```python
from build123d import *

# Parameters (mm, degrees)
F0_W     = 45
F0_H     = 100
F1_DEPTH = 10
F2_W     = 17
F2_H     = 100
F3_DEPTH = 8.5
F4_W     = 34
F4_H     = 100
F5_DEPTH = 7
F8_R     = 16.5
F9_DEPTH = 10


with BuildPart() as f1:
    # F0 (on Top) → F1 (new body)
    with BuildSketch(Plane.XY):
        with Locations((-33.835356, -14.808846)):
            Rectangle(F0_W, F0_H)
    extrude(amount=F1_DEPTH)

    # F2 (on face) → F3 (cut)
    with BuildSketch(Plane.XY.offset(10)):
        with Locations((-33.835356, -14.808846)):
            Rectangle(F2_W, F2_H)
    extrude(amount=-F3_DEPTH, mode=Mode.SUBTRACT)


with BuildPart() as f5:
    # F4 (on Top) → F5 (new body)
    with BuildSketch(Plane.XY):
        with Locations((-39.335356, -14.808846)):
            Rectangle(F4_W, F4_H)
    extrude(amount=F5_DEPTH)


with BuildPart() as f5_1:
    # F6: moved
    add(f5.part.moved(Location((5.5, 0, 1.5))))


with BuildPart() as f1_1:
    add(f1.part)

    # F7: cut F5
    add(f5_1.part, mode=Mode.SUBTRACT)


with BuildPart() as f9:
    # F8 (on Top) → F9 (new body)
    with BuildSketch(Plane.XY):
        with Locations((-33.835356, -64.808846)):
            Circle(F8_R)
    extrude(amount=F9_DEPTH)


with BuildPart() as f9_1:
    # F10: moved
    add(f9.part.moved(Location((0, 50, 4))))


with BuildPart() as f1_2:
    add(f1_1.part)

    # F11: cut F9
    add(f9_1.part, mode=Mode.SUBTRACT)


solid = f1_2.part
```
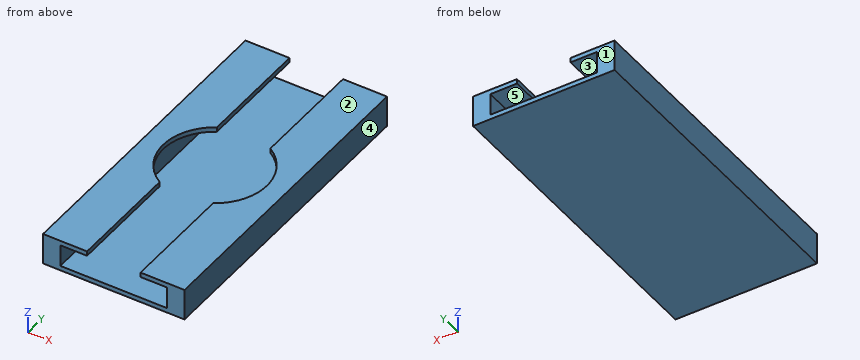
CAD build for the part. Positions are in the model's coordinates, mm. Face numbers are marked on the shaded views. A direction names the side the tool comes from. Coordinates: 2 decimals unless noted, no trailing zeros. Write each loop counter-clockwise with the first axis right and the second up, starting at its lowest first coordinate (ties: lowest second). Pieces come first, ordered by that corner, then holes. Notation, with made-up numbers: (65, -5) -> (86, -5) arc R26 cw to (86, 28) -> close; hole circle Ø4 at (25.5, 30.25). An arc over 180 degrees is marked (long way). Use CSV: the item, a comma, the result in double quotes. Start each with the question number.
Item 1: Band-saw the part on C-C, the plane x = -44. Write the cut outline in (y, z), plus the area to 3 significant figures.
Item 2: Drop a flat-ended pin along its axis: P1, Ø1, axis at x = -33.5, y = -42.5, coming from the +Z side. Give the stop position or say it passes through.
Item 3: Band-saw the part on D-D, the plane x = -23.5. Write the cut outline in (y, z), plus the area to 3 significant figures.
Item 4: Two-plate mould, pull along Z, no slides. Class the marked faces 1, 2 and 3: +Z half, -Z half, draft (parallel to the pull), parting line (faces both ways), or undercut.
Item 5: Band-saw the part on A-A, the plane z = 5.25. Write the cut outline in (x, y).
Item 6: Tool access for the marked faces 4 and 5: list every direction of +Z, -Z, +X, -X, +Y, -Y with a clear straight run to the whole face (end or side of a thin tool).
Item 7: Band-saw the part on B-B, the plane y = -56. Write the cut outline in (x, z), plus the area to 4 significant figures.
Item 8: Wall check: probe 1 along Z at (x, y) = (-20, 20.5); probe 2 along X at (y, z) = (0.5, 6.5); probe 3 along Z at (x, y) = (-35, -15). Give the ranges that are in metal, low to high.
Response values:
1,outline,"(-64.81, 0) -> (35.19, 0) -> (35.19, 1.5) -> (-64.81, 1.5) -> close; (-64.81, 8.5) -> (-27.81, 8.5) -> (-27.81, 10) -> (-64.81, 10) -> close; (-1.81, 8.5) -> (35.19, 8.5) -> (35.19, 10) -> (-1.81, 10) -> close"
1,area,"261 mm2"
2,P1,"stops at z = 1.5"
3,outline,"(-64.81, 0) -> (35.19, 0) -> (35.19, 1.5) -> (-64.81, 1.5) -> close; (-64.81, 8.5) -> (-27.67, 8.5) -> (-27.67, 10) -> (-64.81, 10) -> close; (-1.95, 8.5) -> (35.19, 8.5) -> (35.19, 10) -> (-1.95, 10) -> close"
3,area,"261 mm2"
4,face 1,"draft"
4,face 2,"+Z half"
4,face 3,"undercut"
5,outline,"(-56.34, -64.81) -> (-50.84, -64.81) -> (-50.84, 35.19) -> (-56.34, 35.19) -> close; (-16.84, -64.81) -> (-11.34, -64.81) -> (-11.34, 35.19) -> (-16.84, 35.19) -> close"
6,face 4,"+Z, -Z, +X, +Y, -Y"
6,face 5,"+Y, -Y"
7,outline,"(-56.34, 0) -> (-11.34, 0) -> (-11.34, 10) -> (-25.34, 10) -> (-25.34, 8.5) -> (-16.84, 8.5) -> (-16.84, 1.5) -> (-50.84, 1.5) -> (-50.84, 8.5) -> (-42.34, 8.5) -> (-42.34, 10) -> (-56.34, 10) -> close"
7,area,"186.5 mm2"
8,probe 1,"z = 0 to 1.5, 8.5 to 10"
8,probe 2,"x = -56.34 to -50.84, -16.84 to -11.34"
8,probe 3,"z = 0 to 1.5"
